Part print with two shaded views. Sizes in mm from the minimum x, y, z corner. A direction names the side the tool comes from. Coordinates: 2 decimals unless noted, no trailing zeros. Loops run counter-clockwise (first coordinate to the right, second up) from the corner with the lowest first, then second, coordinate; pieces in that order, holes last. Notation, with made-up numbers: (-4.75, 26) -> (3.25, 26) arc R8 cw to (3.25, 30) -> close; hole circle Ø4 at (65.25, -33). An arc over 180 degrees is marked (long way). Return JSON: item names as keys, results as strings. Group by question number.
(1) Probe L1, parallel to X at y = 16.75, z = 0.45; L2, parallel to X at y = 17.5, z = 2.7; L3, parallel to Y at x = 14.75, z = 2.1. List the from-to ranges inside material, lowest first.
(2) Saw through at D-D on x = 11.5. Write the cut outline in (y, z).
(3) Saw through at A-A on y = 18.75. Write the cut outline in (x, z).
(4) Tool access for the marked faces 1 and 2: list every direction of +Z, -Z, +X, -X, +Y, -Y with a clear straight run to the whole face (end or side of a thin tool).
(5) Flat gauge pins, fed straight in: pin 1 Ø0.6 at (x, z) = (19, 2.5) entering from +Y; pin 2 Ø1.3 at (x, z) = (10.5, 2.5) entering from -Y. Where does each tip first touch, or does it go through?
(6) Mould opens along X. For the marked faces 3 and 4 say: pulls with the +X half, pulls with the -X half, needs draft (parallel to the pull), parting line crosses it, or undercut.
(7) Saw through at B-B on z = 1.45. Write the cut outline in (x, y), then the cut area to 3 significant figures.
(8) Saw through at C-C on y = 5. Write the cut outline in (x, z).
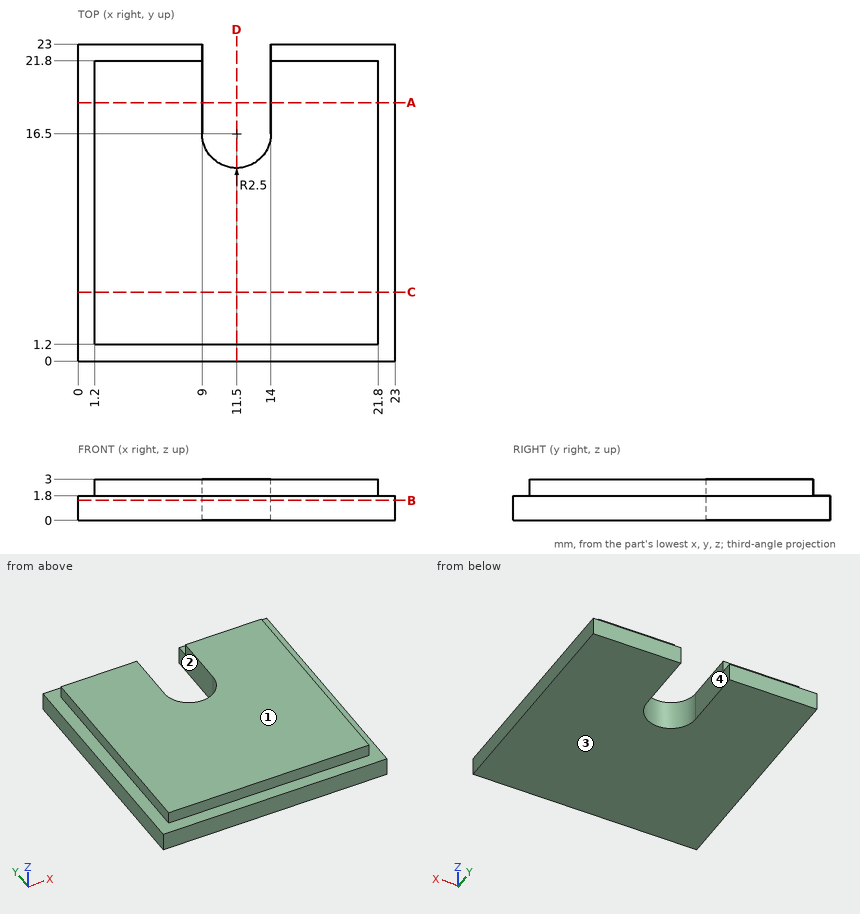
Geometry results:
{
 "1": {"L1": "0 to 9, 14 to 23", "L2": "1.2 to 9, 14 to 21.8", "L3": "1.2 to 21.8"},
 "2": {"outline": "(0, 0) -> (14, 0) -> (14, 3) -> (1.2, 3) -> (1.2, 1.8) -> (0, 1.8) -> close"},
 "3": {"outline": "(0, 0) -> (9, 0) -> (9, 3) -> (1.2, 3) -> (1.2, 1.8) -> (0, 1.8) -> close; (14, 0) -> (23, 0) -> (23, 1.8) -> (21.8, 1.8) -> (21.8, 3) -> (14, 3) -> close"},
 "4": {"face 1": "+Z, +X, -X, +Y, -Y", "face 2": "+Z, -Z, +Y"},
 "5": {"pin 1": "y = 21.8", "pin 2": "y = 1.2"},
 "6": {"face 3": "needs draft", "face 4": "undercut"},
 "7": {"outline": "(0, 0) -> (23, 0) -> (23, 23) -> (14, 23) -> (14, 16.5) arc R2.5 cw to (9, 16.5) -> (9, 23) -> (0, 23) -> close", "area": "487 mm²"},
 "8": {"outline": "(0, 0) -> (23, 0) -> (23, 1.8) -> (21.8, 1.8) -> (21.8, 3) -> (1.2, 3) -> (1.2, 1.8) -> (0, 1.8) -> close"}
}
